from build123d import *

# Parameters (mm, degrees)
SKETCH1_R           = 0.975
BOSS_EXTRUDE1_DEPTH = 23
SKETCH2_W           = 0.95
SKETCH2_H           = 0.95
BOSS_EXTRUDE2_DEPTH = 5
SKETCH3_W           = 1
SKETCH3_H           = 1
CUT_EXTRUDE1_DEPTH  = 5


with BuildPart() as part:
    # Sketch1 → Boss-Extrude1 (new body)
    with BuildSketch(Plane.XY):
        Circle(SKETCH1_R)
    extrude(amount=BOSS_EXTRUDE1_DEPTH)

    # Sketch2 → Boss-Extrude2 (add)
    with BuildSketch(Plane(origin=(0, 0, 0), x_dir=(-1, 0, 0), z_dir=(0, 0, -1))):
        Rectangle(SKETCH2_W, SKETCH2_H)
    extrude(amount=BOSS_EXTRUDE2_DEPTH)

    # Sketch3 → Cut-Extrude1 (cut)
    with BuildSketch(Plane.XY.offset(23)):
        Rectangle(SKETCH3_W, SKETCH3_H)
    extrude(amount=-CUT_EXTRUDE1_DEPTH, mode=Mode.SUBTRACT)


solid = part.part
Design review of the part built by this model. Coordinates are the model's own, in mm. A direction names the side the tool comes from. Coordinates: 2 decimals unless noted, no trailing zeros. Write each loop counter-clockwise with the first axis right and the second up, starting at its lowest first coordinate (ties: lowest second). Pieces come first, ordered by that corner, then holes. Notation, with made-up numbers: (-26.75, -1) - (0.25, -1) arc R31 ccw to (0.25, 35) - close; hole circle Ø6 at (22.5, 85.5). An arc over 180 degrees is marked (long way). Use one line per item in the form item = value.
Q1. For probe 1 along Z at (x, y) = (-0.6, 0.2); probe 2 along Y at (x, z) = (-0.1, 7.5); probe 3 along Z at (x, y) = (0.2, -0.4), list the stretches that pass through material, from the lowest coordinate up.
Taken from the geometry:
probe_1 = 0 to 23
probe_2 = -0.97 to 0.97
probe_3 = -5 to 18
Q2. Machinability: for faces 1 (the flat face through (0, 0, -5)), 2 (the flat face through (-0.475, 0, -2)), 3 (the flat face through (0, 0.475, -2)), 4 (the flat face through (0, 0.5, 21)), which of the approach directions +Z, -Z, +X, -X, +Y, -Y give a long, thin tool a straight path to every point of the face, cutting with its end or side? Answer none if there is none.
Taken from the geometry:
face_1 = -Z, +X, -X, +Y, -Y
face_2 = -Z, -X, +Y, -Y
face_3 = -Z, +X, -X, +Y
face_4 = +Z
Q3. Consider section A-A (z = 21.25). Write out the cut boundary in (x, y) (3 decimals).
Taken from the geometry:
outline = circle Ø1.95 at (0, 0); hole (-0.5, -0.5) - (0.5, -0.5) - (0.5, 0.5) - (-0.5, 0.5) - close
Q4. Insertion check: pin 1 Ø0.5 at (y, z) = (0, -1.5) entering from -X (3 decimals); pin 2 Ø1 at (x, z) = (-0.5, 10) entering from -Y (3 decimals); pin 3 Ø1 at (x, z) = (0, -3.5) entering from +Y (3 decimals); pin 4 Ø0.8 at (y, z) = (0, -2) entering from +X (3 decimals). Each pin has a flat end and moves straight along its axis. Give the tip position at first contact, or say it passes through.
Taken from the geometry:
pin_1 = -0.475
pin_2 = -0.975
pin_3 = 0.475
pin_4 = 0.475
Q5. The part is to be moulded in two halves that separate along X. For faces 5 (the flat face through (0, -0.475, -2)), 6 (the flat face through (0.475, 0, -2)), 7 (the flat face through (0.5, 0, 21)), 8 (the cylindrical face through (-0.72, 0.66, 11.34)), say which applies: +X half, -X half, draft (parallel to the pull), parting line (faces both ways), or undercut.
Taken from the geometry:
face_5 = draft
face_6 = +X half
face_7 = undercut
face_8 = parting line
Q6. Consider section B-B (x = 0). Write out the cut boundary in (y, z) (3 decimals).
Taken from the geometry:
outline = (-0.975, 0) - (-0.475, 0) - (-0.475, -5) - (0.475, -5) - (0.475, 0) - (0.975, 0) - (0.975, 23) - (0.5, 23) - (0.5, 18) - (-0.5, 18) - (-0.5, 23) - (-0.975, 23) - close
Q7. Consider section D-D (z = -1.75). Write out the cut boundary in (x, y) (3 decimals).
Taken from the geometry:
outline = (-0.475, -0.475) - (0.475, -0.475) - (0.475, 0.475) - (-0.475, 0.475) - close
